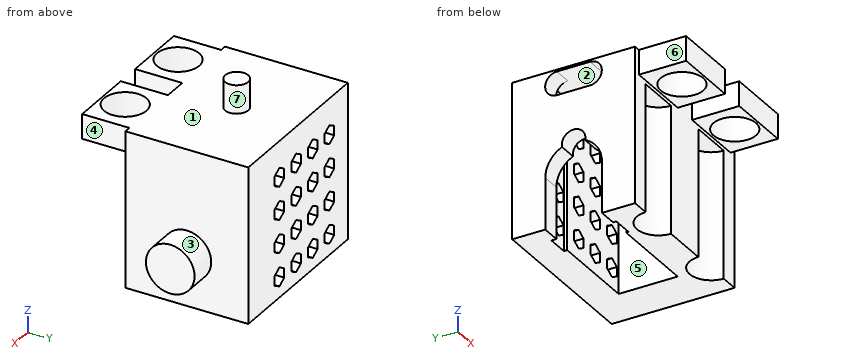
from build123d import *

# Parameters (mm, degrees)
SKETCH007_W          = 35.81
SKETCH007_H          = 26
PAD002_DEPTH         = 33
SKETCH008_R          = 2.45
PAD003_DEPTH         = 6
SKETCH009_W          = 13.978334
SKETCH009_H          = 5.221016
SKETCH009_W_2        = 13.87282
PAD004_DEPTH         = 10
SKETCH010_R          = 4.5
POCKET_DEPTH         = 11.222016
SKETCH016_W          = 22.6
SKETCH016_H          = 12.5
POCKET004_DEPTH      = 27.6
POCKET005_DEPTH      = 5.4
SKETCH018_W          = 4.8
SKETCH018_H          = 12
POCKET006_DEPTH      = 5
POCKET007_DEPTH      = 8.5
POCKET008_DEPTH      = 200
POCKET008_DEPTH_BACK = 200
POCKET036_DEPTH      = 5
SKETCH099_R          = 5.15
PAD045_DEPTH         = 6
SKETCH100_W          = 4.510635
SKETCH100_H          = 13.729386
POCKET046_DEPTH      = 34
POCKET047_DEPTH      = 9
POCKET048_DEPTH      = 27


with BuildPart() as part:
    # Sketch007 → Pad002 (new body)
    with BuildSketch(Plane.XY):
        with Locations((52.505, 52.5)):
            Rectangle(SKETCH007_W, SKETCH007_H)
    extrude(amount=PAD002_DEPTH)

    # Sketch008 (on Face6 of Pad002) → Pad003 (join)
    with BuildSketch(Plane.XY.offset(33)):
        with Locations((52.5, 52.5)):
            Circle(SKETCH008_R)
    extrude(amount=PAD003_DEPTH)

    # Sketch009 (on Face1 of Pad003) → Pad004 (join)
    with BuildSketch(Plane.XZ.offset(-39.5)):
        with Locations((42.979167, 30.389492)):
            Rectangle(SKETCH009_W, SKETCH009_H)
        with Locations((62.05359, 30.389492)):
            Rectangle(SKETCH009_W_2, SKETCH009_H)
    extrude(amount=PAD004_DEPTH)

    # Sketch010 (on Face6 of Pad004) → Pocket (cut, through all)
    with BuildSketch(Plane(origin=(0, 0, 27.778984), x_dir=(1, 0, 0), z_dir=(0, 0, -1))):
        with Locations((62, -34.5)):
            Circle(SKETCH010_R)
        with Locations((43, -34.5)):
            Circle(SKETCH010_R)
    extrude(amount=-POCKET_DEPTH, mode=Mode.SUBTRACT)

    # Sketch016 → Pocket004 (cut)
    with BuildSketch(Plane(origin=(0, 0, 0), x_dir=(1, 0, 0), z_dir=(0, 0, -1))):
        with Locations((50.3, -52.6)):
            Rectangle(SKETCH016_W, SKETCH016_H)
    extrude(amount=-POCKET004_DEPTH, mode=Mode.SUBTRACT)

    # Sketch015 (on Face3 of Pocket) → Pocket005 (cut)
    with BuildSketch(Plane(origin=(34.6, 0, 0), x_dir=(0, -1, 0), z_dir=(-1, 0, 0))):
        with BuildLine():
            Line((-58.5, 0), (-46.5, 0))
            Line((-46.5, 0), (-46.5, 10.9))
            ThreePointArc((-46.5, 10.9), (-47.4637930268, 14.1613830383), (-50.0455397742, 16.375))
            ThreePointArc((-50.0455397742, 16.375), (-52.5, 19.35), (-54.9544602258, 16.375))
            ThreePointArc((-54.9544602258, 16.375), (-57.5362069732, 14.1613830383), (-58.5, 10.9))
            Line((-58.5, 10.9), (-58.5, 0))
        make_face()
    extrude(amount=-POCKET005_DEPTH, mode=Mode.SUBTRACT)

    # Sketch018 → Pocket006 (cut)
    with BuildSketch(Plane(origin=(0, 0, 27.6), x_dir=(1, 0, 0), z_dir=(0, 0, -1))):
        with Locations((43.6, -52.5)):
            Rectangle(SKETCH018_W, SKETCH018_H)
    extrude(amount=-POCKET006_DEPTH, mode=Mode.SUBTRACT)

    # Sketch020 (on Face3 of Pocket006) → Pocket007 (cut)
    with BuildSketch(Plane(origin=(34.6, 0, 0), x_dir=(0, -1, 0), z_dir=(-1, 0, 0))):
        with BuildLine():
            ThreePointArc((-56.04, 32.6), (-58.53, 30.11), (-56.04, 27.62))
            Line((-56.04, 27.62), (-49.02, 27.62))
            ThreePointArc((-49.02, 27.62), (-46.53, 30.11), (-49.02, 32.6))
            Line((-56.04, 32.6), (-49.02, 32.6))
        make_face()
    extrude(amount=-POCKET007_DEPTH, mode=Mode.SUBTRACT)

    # Sketch021 (on Face9 of Pocket007) → Pocket008 (cut, two sides)
    with BuildSketch(Plane(origin=(0, 0, 27.778984), x_dir=(1, 0, 0), z_dir=(0, 0, -1))) as pocket008_sk:
        Polygon((-57.6610266203, 24.8205080757), (-59.6610266203, 25.9752086141), (-61.6610266203, 24.8205080757), (-61.6610266203, 22.5111069989), (-59.6610266203, 21.3564064606), (-57.6610266203, 22.5111069989), align=None)
        Polygon((-57.6610266203, 18.2017059222), (-59.6610266203, 19.3564064606), (-61.6610266203, 18.2017059222), (-61.6610266203, 15.8923048454), (-59.6610266203, 14.737604307), (-57.6610266203, 15.8923048454), align=None)
        Polygon((-57.6610266203, 11.5829037687), (-59.6610266203, 12.737604307), (-61.6610266203, 11.5829037687), (-61.6610266203, 9.2735026919), (-59.6610266203, 8.1188021535), (-57.6610266203, 9.2735026919), align=None)
        Polygon((-57.6610266203, 4.9641016151), (-59.6610266203, 6.1188021535), (-61.6610266203, 4.9641016151), (-61.6610266203, 2.6547005384), (-59.6610266203, 1.5), (-57.6610266203, 2.6547005384), align=None)
        Polygon((-45.6610266203, 24.8205080757), (-47.6610266203, 25.9752086141), (-49.6610266203, 24.8205080757), (-49.6610266203, 22.5111069989), (-47.6610266203, 21.3564064606), (-45.6610266203, 22.5111069989), align=None)
        Polygon((-45.6610266203, 18.2017059222), (-47.6610266203, 19.3564064606), (-49.6610266203, 18.2017059222), (-49.6610266203, 15.8923048454), (-47.6610266203, 14.737604307), (-45.6610266203, 15.8923048454), align=None)
        Polygon((-45.6610266203, 11.5829037687), (-47.6610266203, 12.737604307), (-49.6610266203, 11.5829037687), (-49.6610266203, 9.2735026919), (-47.6610266203, 8.1188021535), (-45.6610266203, 9.2735026919), align=None)
        Polygon((-45.6610266203, 4.9641016151), (-47.6610266203, 6.1188021535), (-49.6610266203, 4.9641016151), (-49.6610266203, 2.6547005384), (-47.6610266203, 1.5), (-45.6610266203, 2.6547005384), align=None)
        Polygon((-39.6610266203, 24.8205080757), (-41.6610266203, 25.9752086141), (-43.6610266203, 24.8205080757), (-43.6610266203, 22.5111069989), (-41.6610266203, 21.3564064606), (-39.6610266203, 22.5111069989), align=None)
        Polygon((-39.6610266203, 18.2017059222), (-41.6610266203, 19.3564064606), (-43.6610266203, 18.2017059222), (-43.6610266203, 15.8923048454), (-41.6610266203, 14.737604307), (-39.6610266203, 15.8923048454), align=None)
        Polygon((-39.6610266203, 11.5829037687), (-41.6610266203, 12.737604307), (-43.6610266203, 11.5829037687), (-43.6610266203, 9.2735026919), (-41.6610266203, 8.1188021535), (-39.6610266203, 9.2735026919), align=None)
        Polygon((-39.6610266203, 4.9641016151), (-41.6610266203, 6.1188021535), (-43.6610266203, 4.9641016151), (-43.6610266203, 2.6547005384), (-41.6610266203, 1.5), (-39.6610266203, 2.6547005384), align=None)
        Polygon((-51.6610266203, 24.8205080757), (-53.6610266203, 25.9752086141), (-55.6610266203, 24.8205080757), (-55.6610266203, 22.5111069989), (-53.6610266203, 21.3564064606), (-51.6610266203, 22.5111069989), align=None)
        Polygon((-51.6610266203, 18.2017059222), (-53.6610266203, 19.3564064606), (-55.6610266203, 18.2017059222), (-55.6610266203, 15.8923048454), (-53.6610266203, 14.737604307), (-51.6610266203, 15.8923048454), align=None)
        Polygon((-51.6610266203, 11.5829037687), (-53.6610266203, 12.737604307), (-55.6610266203, 11.5829037687), (-55.6610266203, 9.2735026919), (-53.6610266203, 8.1188021535), (-51.6610266203, 9.2735026919), align=None)
        Polygon((-51.6610266203, 4.9641016151), (-53.6610266203, 6.1188021535), (-55.6610266203, 4.9641016151), (-55.6610266203, 2.6547005384), (-53.6610266203, 1.5), (-51.6610266203, 2.6547005384), align=None)
    extrude(amount=-POCKET008_DEPTH, mode=Mode.SUBTRACT)
    extrude(pocket008_sk.sketch, amount=POCKET008_DEPTH_BACK, mode=Mode.SUBTRACT)

    # CopySketch077 → Pocket036 (cut)
    with BuildSketch(Plane.XZ.offset(10)):
        with BuildLine():
            ThreePointArc((49.5809685833, -52.61365544), (52.5285478813, -63.912849758), (55.405181515, -52.5953856034))
            ThreePointArc((55.405181515, -52.5953856034), (52.4814034168, -48.8837389355), (49.5809685833, -52.61365544))
        make_face()
    extrude(amount=-POCKET036_DEPTH, mode=Mode.SUBTRACT)

    # Sketch099 (on Face11 of Pocket036) → Pad045 (join)
    with BuildSketch(Plane.YZ.offset(70.41)):
        with Locations((52.5, 10.752384)):
            Circle(SKETCH099_R)
    extrude(amount=PAD045_DEPTH)

    # Sketch100 (on Face44 of Pad045) → Pocket046 (cut)
    with BuildSketch(Plane(origin=(0, 0, 32.6), x_dir=(1, 0, 0), z_dir=(0, 0, -1))):
        with Locations((40.8446805, -52.688568)):
            Rectangle(SKETCH100_W, SKETCH100_H)
    extrude(amount=POCKET046_DEPTH, mode=Mode.SUBTRACT)

    # Sketch101 (on Face12 of Pocket046) → Pocket047 (cut)
    with BuildSketch(Plane(origin=(0, 65.5, 0), x_dir=(-1, 0, 0), z_dir=(0, 1, 0))):
        Polygon((-59.214752, 23.341819945), (-57.4827011924, 24.341819945), (-57.4827011924, 26.341819945), (-59.214752, 27.341819945), (-60.9468028076, 26.341819945), (-60.9468028076, 24.341819945), align=None)
        Polygon((-59.214752, 16.341819945), (-57.4827011924, 17.341819945), (-57.4827011924, 19.341819945), (-59.214752, 20.341819945), (-60.9468028076, 19.341819945), (-60.9468028076, 17.341819945), align=None)
        Polygon((-59.214752, 9.341819945), (-57.4827011924, 10.341819945), (-57.4827011924, 12.341819945), (-59.214752, 13.341819945), (-60.9468028076, 12.341819945), (-60.9468028076, 10.341819945), align=None)
        Polygon((-59.214752, 2.341819945), (-57.4827011924, 3.341819945), (-57.4827011924, 5.341819945), (-59.214752, 6.341819945), (-60.9468028076, 5.341819945), (-60.9468028076, 3.341819945), align=None)
        Polygon((-53.214752, 23.341819945), (-51.4827011924, 24.341819945), (-51.4827011924, 26.341819945), (-53.214752, 27.341819945), (-54.9468028076, 26.341819945), (-54.9468028076, 24.341819945), align=None)
        Polygon((-53.214752, 16.341819945), (-51.4827011924, 17.341819945), (-51.4827011924, 19.341819945), (-53.214752, 20.341819945), (-54.9468028076, 19.341819945), (-54.9468028076, 17.341819945), align=None)
        Polygon((-53.214752, 9.341819945), (-51.4827011924, 10.341819945), (-51.4827011924, 12.341819945), (-53.214752, 13.341819945), (-54.9468028076, 12.341819945), (-54.9468028076, 10.341819945), align=None)
        Polygon((-53.214752, 2.341819945), (-51.4827011924, 3.341819945), (-51.4827011924, 5.341819945), (-53.214752, 6.341819945), (-54.9468028076, 5.341819945), (-54.9468028076, 3.341819945), align=None)
        Polygon((-47.214752, 23.364838), (-45.4827011924, 24.364838), (-45.4827011924, 26.364838), (-47.214752, 27.364838), (-48.9468028076, 26.364838), (-48.9468028076, 24.364838), align=None)
        Polygon((-47.214752, 16.364838), (-45.4827011924, 17.364838), (-45.4827011924, 19.364838), (-47.214752, 20.364838), (-48.9468028076, 19.364838), (-48.9468028076, 17.364838), align=None)
        Polygon((-47.214752, 9.364838), (-45.4827011924, 10.364838), (-45.4827011924, 12.364838), (-47.214752, 13.364838), (-48.9468028076, 12.364838), (-48.9468028076, 10.364838), align=None)
        Polygon((-47.214752, 2.364838), (-45.4827011924, 3.364838), (-45.4827011924, 5.364838), (-47.214752, 6.364838), (-48.9468028076, 5.364838), (-48.9468028076, 3.364838), align=None)
        Polygon((-41.214752, 23.364838), (-39.4827011924, 24.364838), (-39.4827011924, 26.364838), (-41.214752, 27.364838), (-42.9468028076, 26.364838), (-42.9468028076, 24.364838), align=None)
        Polygon((-41.214752, 16.364838), (-39.4827011924, 17.364838), (-39.4827011924, 19.364838), (-41.214752, 20.364838), (-42.9468028076, 19.364838), (-42.9468028076, 17.364838), align=None)
        Polygon((-41.214752, 9.364838), (-39.4827011924, 10.364838), (-39.4827011924, 12.364838), (-41.214752, 13.364838), (-42.9468028076, 12.364838), (-42.9468028076, 10.364838), align=None)
        Polygon((-41.214752, 2.364838), (-39.4827011924, 3.364838), (-39.4827011924, 5.364838), (-41.214752, 6.364838), (-42.9468028076, 5.364838), (-42.9468028076, 3.364838), align=None)
    extrude(amount=-POCKET047_DEPTH, mode=Mode.SUBTRACT)

    # Sketch102 (on Face2 of Pocket047) → Pocket048 (cut)
    with BuildSketch(Plane(origin=(0, 0, 0), x_dir=(1, 0, 0), z_dir=(0, 0, -1))):
        with BuildLine():
            ThreePointArc((47.558878, -33.45), (42.978878, -28.87), (38.398878, -33.45))
            Line((38.398878, -33.45), (38.398878, -39.45))
            ThreePointArc((38.398878, -39.45), (42.978878, -44.03), (47.558878, -39.45))
            Line((47.558878, -33.45), (47.558878, -39.45))
        make_face()
        with BuildLine():
            ThreePointArc((66.5366215742, -33.45), (61.9566215742, -28.87), (57.3766215742, -33.45))
            Line((57.3766215742, -33.45), (57.3766215742, -39.45))
            ThreePointArc((57.3766215742, -39.45), (61.9566215742, -44.03), (66.5366215742, -39.45))
            Line((66.5366215742, -33.45), (66.5366215742, -39.45))
        make_face()
    extrude(amount=-POCKET048_DEPTH, mode=Mode.SUBTRACT)


with BuildPart() as part_1:
    # Body002 placement: moved
    add(part.part.moved(Location((0, 0, -55))))


solid = part_1.part
For this review, take the finished solid that the model builds, in its own axes (mm). Face numbers are marked on the shaded views. A direction names the side the tool comes from. Round coordinates to 2 decimals unless told otherwise and drop trailing zeros. Order: outer loops, then holes, each group sorted by start corner. A loop starts at its lowest first (then second) coordinate and runs counter-clockwise, first axis right, second up. Notation, with made-up numbers: (-23.5, -7) -> (13.5, -7) arc R22 ccw to (13.5, 23) -> close; hole circle Ø4 at (38, 32). An arc over 180 degrees is marked (long way). Put each result on its own line as item: value.
Q1. Add section B-B on x = 52.5. Write out the cut boundary in (y, z), plus the area to 3 significant figures.
Check result:
outline: (39.5, -55) -> (46.35, -55) -> (46.35, -27.4) -> (58.85, -27.4) -> (58.85, -28.07) -> (65.5, -28.07) -> (65.5, -22) -> (54.95, -22) -> (54.95, -16) -> (50.05, -16) -> (50.05, -22) -> (39.5, -22) -> close; (58.85, -55) -> (65.5, -55) -> (65.5, -52.25) -> (58.85, -52.25) -> close; (58.85, -49.07) -> (65.5, -49.07) -> (65.5, -45.25) -> (58.85, -45.25) -> close; (58.85, -42.07) -> (65.5, -42.07) -> (65.5, -38.25) -> (58.85, -38.25) -> close; (58.85, -35.07) -> (65.5, -35.07) -> (65.5, -31.25) -> (58.85, -31.25) -> close
area: 458 mm2
Q2. Insertion check: pin 1 Ø16.5 at (x, z) = (49, -42.5) entering from -Y; pin 2 Ø0.6 at (y, z) = (63.5, -36.5) entering from +X; pin 3 Ø10 at (x, y) = (49.5, 52.5) entering from -Z; pin 4 Ø1.4 at (x, z) = (40.5, -31) entering from +Y. Each pin has a flat end and moves straight along its axis. Give the tip position at first contact, or say it passes through.
Check result:
pin 1: y = 39.5
pin 2: x = 70.41
pin 3: z = -27.4
pin 4: y = 65.5
Q3. Add section D-D on z = -19. Write out the cut boundary in (x, y).
Check result:
outline: circle Ø4.9 at (52.5, 52.5)
Q4. Add section A-A on y = 34.5. Write out the cut boundary in (x, z).
Check result:
outline: (35.99, -27.22) -> (38.5, -27.22) -> (38.5, -22) -> (35.99, -22) -> close; (47.5, -27.22) -> (49.97, -27.22) -> (49.97, -22) -> (47.5, -22) -> close; (55.12, -27.22) -> (57.5, -27.22) -> (57.5, -22) -> (55.12, -22) -> close; (66.5, -27.22) -> (68.99, -27.22) -> (68.99, -22) -> (66.5, -22) -> close
Q5. Machinability: for the marked faces 4, 5, 6 and 7, which of the approach directions +Z, -Z, +X, -X, +Y, -Y give a long, thin tool a straight path to every point of the face, cutting with its end or side? Answer none if there is none.
Check result:
face 4: +Z, -Z, +X, -Y
face 5: -Z
face 6: +Z, -Z, -X, -Y
face 7: +Z
Q6. Add section C-C on x = 58.5. State how many separate pieces and enclosed holes the cut face has, plus the area to 3 significant figures.
Check result:
separate pieces: 6
enclosed holes: 0
area: 371 mm2
Q7. Mouldability with a two-part tool opening along Y and no side actions: class the marked faces 1, 2 and 3 as pulls with the +Y half, pulls with the -Y half, needs draft (parallel to the pull), parting line crosses it, or undercut.
Check result:
face 1: needs draft
face 2: undercut
face 3: parting line crosses it
Q8. For probe 1 along Y at (x, z) = (43, -23.2); probe 2 along X at (y, z) = (57, -32); probe 3 along Z at (x, y) = (37, 52.5), list the stretches that pass through material, from the lowest coordinate up. Write a range as [from, to].
Check result:
probe 1: [29.5, 30], [39, 45.82], [59.55, 65.5]
probe 2: [34.6, 38.59], [61.6, 70.41]
probe 3: [-35.65, -27.38], [-22.4, -22]
